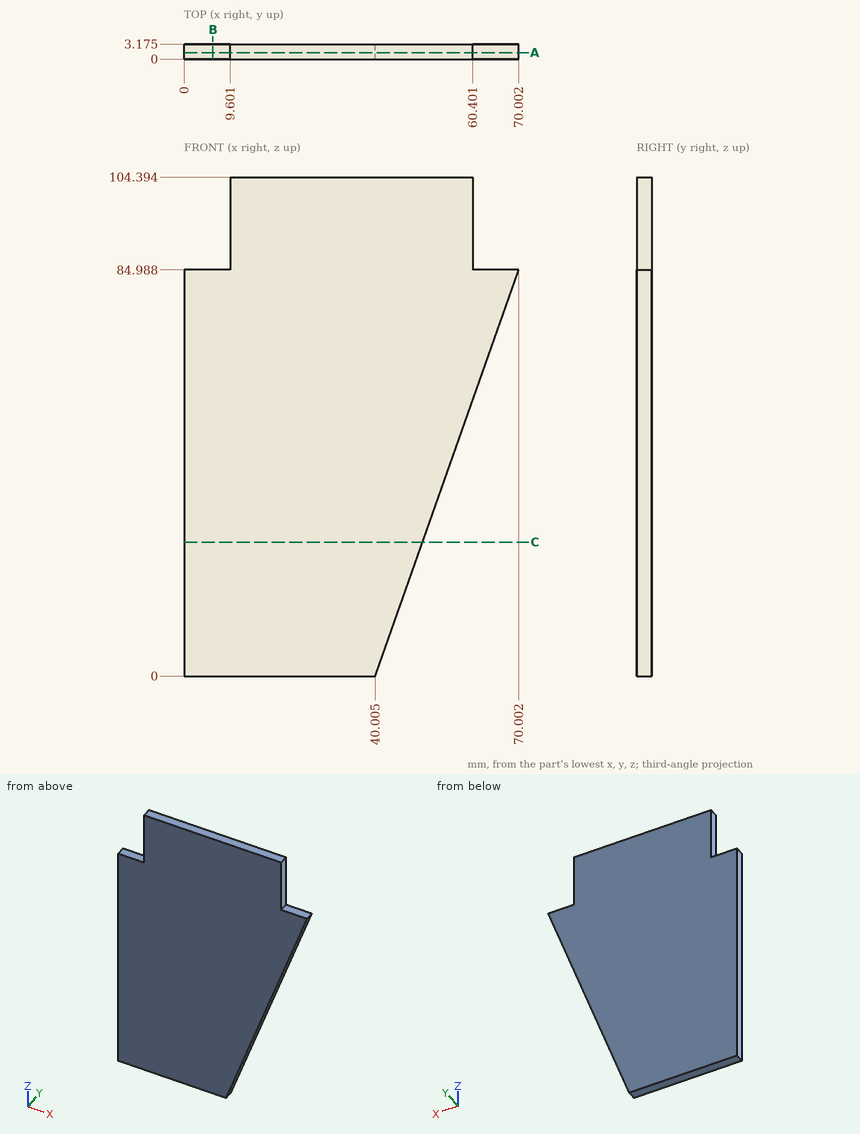
Verification items for this drawing (mm, ordinates from the low corner). Coordinates: 2 decimals unless noted, no trailing zeros. Write each loop counter-clockwise with the first axis right and the second up, starting at its lowest first coordinate (ties: lowest second). Pieces come first, ordered by that corner, then holes. Notation, with made-up numbers: M -10.5,-24 L -2.5,-24 A15 cw -2.5,-15 Z; hole C -34,49.5 d6. An arc over 180 degrees is marked long. Answer as a JSON object with one key per item and string values.
1. Section check A-A, the plane y = 1.35. Enter the section's corners in (x, z) (1 decimal).
Answers below:
{"outline": "M 0,0 L 40,0 L 70,85 L 60.4,85 L 60.4,104.4 L 9.6,104.4 L 9.6,85 L 0,85 Z"}
2. Go/stop test with flat-tipped pins: pin 1 Ø1.5 at (y, z) = (2.5, 28.5) entering from +X; pin 2 Ø1.6 at (x, y) = (5.5, 1) entering from +Z. Record where each tip stops, or that it passes through.
Answers below:
{"pin 1": "stops at x = 50.33", "pin 2": "stops at z = 84.99"}
3. Section check B-B, the plane x = 6. Enter the section's corners in (y, z) (1 decimal).
Answers below:
{"outline": "M 0,0 L 3.2,0 L 3.2,85 L 0,85 Z"}
4. Section check C-C, the plane z = 28. Enter the section's corners in (x, y) (1 decimal), plus the area to 3 significant figures.
Answers below:
{"outline": "M 0,0 L 49.9,0 L 49.9,3.2 L 0,3.2 Z", "area": "158 mm²"}
5. Scan lines: L1, parallel to Z at x = 9, y = 2.3; L2, parallel to X at y = 2.65, z = 90; L3, parallel to X at y = 1, z = 81.5. Record each from-to range of solid material in increasing order.
Answers below:
{"L1": "z = 0 to 84.99", "L2": "x = 9.6 to 60.4", "L3": "x = 0 to 68.77"}
